Verification items for the finished model (mm, model axes). A direction names the side the tool comes from. Round coordinates to 2 decimals unless told otherwise and drop trailing zeros. Loops run counter-clockwise (first coordinate to the right, second up) from the corner with the lowest first, then second, coordinate; pieces in that order, holes last. Notation, with made-up numbers: (74.25, 53) -> (81.25, 53) arc R12 ccw to (81.25, 68) -> close; hole circle Ø9 at (44.25, 68.25). An arc over 180 degrees is marked (long way). Use CSV: the item, a comma, the result in double quotes. Start each with the question number.
```python
from build123d import *

# Parameters (mm, degrees)
SKETCH_1_W          = 30
SKETCH_1_H          = 65
EXTRUDE_1_DEPTH     = 48
SKETCH_2_W          = 30
SKETCH_2_H          = 82
EXTRUDE_2_DEPTH     = 4
SKETCH_3_R          = 2.7
CUT_EXTRUDE_1_DEPTH = 4
SKETCH_4_R          = 4
EXTRUDE_3_DEPTH     = 7
CHAMFER_1_SIZE      = 0.3
FILLET_1_R          = 2
CHAMFER_2_SIZE      = 5
FILLET_2_R          = 2


with BuildPart() as part:
    # 草图1 → 凸台-拉伸1 (new body)
    with BuildSketch(Plane(origin=(0, 0, 0), x_dir=(1, 0, 0), z_dir=(0, 1, 0))):
        Rectangle(SKETCH_1_W, SKETCH_1_H)
    extrude(amount=EXTRUDE_1_DEPTH)

    # 草图2 → 凸台-拉伸2 (add)
    with BuildSketch(Plane(origin=(0, 35.5, 0), x_dir=(-1, 0, 0), z_dir=(0, -1, 0))):
        Rectangle(SKETCH_2_W, SKETCH_2_H)
    extrude(amount=EXTRUDE_2_DEPTH)

    # 草图3 → 切除-拉伸1 (cut)
    with BuildSketch(Plane(origin=(0, 35.5, 0), x_dir=(1, 0, 0), z_dir=(0, 1, 0))):
        with Locations(Location((-8.25, 37.5, 0), (0, 0, 270))):
            Circle(SKETCH_3_R)
        with Locations(Location((8.25, 37.5, 0), (0, 0, 270))):
            Circle(SKETCH_3_R)
        with Locations(Location((8.25, -37.5, 0), (0, 0, 270))):
            Circle(SKETCH_3_R)
        with Locations(Location((-8.25, -37.5, 0), (0, 0, 270))):
            Circle(SKETCH_3_R)
    extrude(amount=-CUT_EXTRUDE_1_DEPTH, mode=Mode.SUBTRACT)

    # 草图4 → 凸台-拉伸3 (add)
    with BuildSketch(Plane(origin=(0, 48, 0), x_dir=(1, 0, 0), z_dir=(0, 1, 0))):
        with Locations(Location((0, 19.5, 0), (0, 0, 90))):
            Circle(SKETCH_4_R)
    extrude(amount=EXTRUDE_3_DEPTH)

    # 倒角1
    chamfer_1_edges = [part.edges().sort_by_distance(p)[0] for p in [
        (0, 55, -15.5),
    ]]
    chamfer(chamfer_1_edges, length=CHAMFER_1_SIZE)

    # 圆角1
    fillet_1_edges = [part.edges().sort_by_distance(p)[0] for p in [
        (15, 15.75, 32.5),
        (-15, 15.75, 32.5),
        (-15, 15.75, -32.5),
        (15, 15.75, -32.5),
        (15, 41.75, 32.5),
        (-15, 41.75, 32.5),
    ]]
    fillet(fillet_1_edges, radius=FILLET_1_R)

    # 倒角2
    chamfer_2_edges = [part.edges().sort_by_distance(p)[0] for p in [
        (0, 48, -32.5),
    ]]
    chamfer(chamfer_2_edges, length=CHAMFER_2_SIZE)

    # 圆角2
    fillet_2_edges = [part.edges().sort_by_distance(p)[0] for p in [
        (-15, 39.25, -32.5),
        (15, 39.25, -32.5),
        (15, 33.5, -41),
        (-15, 33.5, 41),
        (15, 33.5, 41),
        (-15, 33.5, -41),
    ]]
    fillet(fillet_2_edges, radius=FILLET_2_R)


solid = part.part
```
Q1. Cross-section at A-A (x = 8.25). Record the boundary of the cut face in (y, z).
Q2. Thickness scan on L1, parallel to X at y = 34.2, z = -37.5; L2, parallel to Z at x = -10.5, y = 5.5; L3, parallel to Y at x = -6.75, z = -19. Record the ranges inside material, lowest first. Write a range as from..to.
Q3. Cross-section at B-B (z = 37.5). Record the boundary of the cut face in (x, y), and give its area (3 significant figures).
Q4. Tool access check on faces 1 (the face through (-14.43, 15.97, 31.9)), 2 (the face through (0, 42, 32.5)), 3 (the face through (0, 39, -32.5)). Record the directions out of +Z, -Z, +X, -X, +Y, -Y that give a thin tool (end or side, any length) a straight path to the whole face; none if there is none.
Q5. Cross-section at D-D (x = 0). Record the boundary of the cut face in (y, z).
Q6. Cross-section at C-C (y = 34). Record the boundary of the cut face in (x, z), and give its area (3 significant figures).
Q7. Depth check by flat-ended pin: pin 1 Ø11.5 at (x, z) = (-7, 35) entering from +Y; pin 2 Ø6 at (x, y) = (-3, 43) entering from +Z; pin 3 Ø8.5 at (x, z) = (8.25, -37.5) entering from -Y; pin 4 Ø3 at (x, z) = (8.25, 37.5) entering from +Y. Enter the tip coordinate at first touch or a pass-through.
Q8. Release check for a two-part mould opening along X. For faces 4 (the face through (0, 16, -32.5)), 5 (the face through (-14.43, 41.84, 31.9)), 6 (the face through (-7.439, 33.528, 40.075)) record: +X half, -X half, draft (parallel to the pull), parting line (faces both ways), or undercut.
Answer list:
1,outline,"(0, -32.5) -> (31.5, -32.5) -> (31.5, -34.8) -> (35.5, -34.8) -> (35.5, -32.5) -> (43, -32.5) -> (48, -27.5) -> (48, 32.5) -> (35.5, 32.5) -> (35.5, 34.8) -> (31.5, 34.8) -> (31.5, 32.5) -> (0, 32.5) -> close; (31.5, -41) -> (35.5, -41) -> (35.5, -40.2) -> (31.5, -40.2) -> close; (31.5, 40.2) -> (35.5, 40.2) -> (35.5, 41) -> (31.5, 41) -> close"
2,L1,"x = -15..-10.95, -5.55..5.55, 10.95..15"
2,L2,"z = -32.5..32.5"
2,L3,"y = 0..48"
3,outline,"(-15, 31.5) -> (-10.95, 31.5) -> (-10.95, 35.5) -> (-15, 35.5) -> close; (-5.55, 31.5) -> (5.55, 31.5) -> (5.55, 35.5) -> (-5.55, 35.5) -> close; (10.95, 31.5) -> (15, 31.5) -> (15, 35.5) -> (10.95, 35.5) -> close"
3,area,"76.8 mm2"
4,face 1,"+Z, -X, -Y"
4,face 2,"+Z, +X, -X, +Y"
4,face 3,"-Z, +X, -X, +Y"
5,outline,"(0, -32.5) -> (31.5, -32.5) -> (31.5, -41) -> (35.5, -41) -> (35.5, -32.5) -> (43, -32.5) -> (48, -27.5) -> (48, -23.5) -> (54.7, -23.5) -> (55, -23.2) -> (55, -15.8) -> (54.7, -15.5) -> (48, -15.5) -> (48, 32.5) -> (35.5, 32.5) -> (35.5, 41) -> (31.5, 41) -> (31.5, 32.5) -> (0, 32.5) -> close"
6,outline,"(-15, -39) arc R2 ccw to (-13, -41) -> (13, -41) arc R2 ccw to (15, -39) -> (15, 39) arc R2 ccw to (13, 41) -> (-13, 41) arc R2 ccw to (-15, 39) -> close; hole circle Ø5.4 at (-8.25, -37.5); hole circle Ø5.4 at (-8.25, 37.5); hole circle Ø5.4 at (8.25, -37.5); hole circle Ø5.4 at (8.25, 37.5)"
6,area,"2,360 mm2"
7,pin 1,"stops at y = 48"
7,pin 2,"stops at z = 32.5"
7,pin 3,"stops at y = 31.5"
7,pin 4,"passes through"
8,face 4,"draft"
8,face 5,"-X half"
8,face 6,"undercut"
